```python
from build123d import *

# Parameters (mm, degrees)
CYLINDER001_R              = 1.5
CYLINDER001_DEPTH          = 10
BOX001_W                   = 5
BOX001_H                   = 2
BOX001_DEPTH               = 5
BOX_W                      = 5
BOX_H                      = 5
BOX_DEPTH                  = 10
FILLET_R                   = 2
FILLET_PLACEMENT_ANGLE     = 90
CHAMFER_SIZE               = 4
SKETCH005_R                = 54
SKETCH005_R_2              = 48.75
PAD003_DEPTH               = 1.5
SKETCH006_R                = 1.5
POCKET002_DEPTH            = 1.501
CYLINDER003_R              = 1.5
CYLINDER003_DEPTH          = 10
BOX005_W                   = 5
BOX005_H                   = 2
BOX005_DEPTH               = 5
BOX004_W                   = 5
BOX004_H                   = 5
BOX004_DEPTH               = 10
FILLET002_R                = 2
FILLET002_PLACEMENT_ANGLE  = 90
CHAMFER002_SIZE            = 4
CHAMFER002_PLACEMENT_ANGLE = 90
CYLINDER004_R              = 1.5
CYLINDER004_DEPTH          = 10
BOX007_W                   = 5
BOX007_H                   = 2
BOX007_DEPTH               = 5
BOX006_W                   = 5
BOX006_H                   = 5
BOX006_DEPTH               = 10
FILLET003_R                = 2
FILLET003_PLACEMENT_ANGLE  = 90
CHAMFER003_SIZE            = 4
CHAMFER003_PLACEMENT_ANGLE = 180
CYLINDER005_R              = 1.5
CYLINDER005_DEPTH          = 10
BOX009_W                   = 5
BOX009_H                   = 2
BOX009_DEPTH               = 5
BOX008_W                   = 5
BOX008_H                   = 5
BOX008_DEPTH               = 10
FILLET004_R                = 2
FILLET004_PLACEMENT_ANGLE  = 90
CHAMFER004_SIZE            = 4
CHAMFER004_PLACEMENT_ANGLE = 90


with BuildPart() as screw:
    # Cylinder001 → Cylinder001 (new body)
    with BuildSketch(Plane(origin=(2.5, -2.75, 7.5), x_dir=(0, 0, 1), z_dir=(0, 1, 0))):
        Circle(CYLINDER001_R)
    extrude(amount=CYLINDER001_DEPTH)


with BuildPart() as extleghole:
    # Box001 → Box001 (new body)
    with BuildSketch(Plane(origin=(0, 1.5, 5), x_dir=(1, 0, 0), z_dir=(0, 0, 1))):
        with Locations((2.5, 1)):
            Rectangle(BOX001_W, BOX001_H)
    extrude(amount=BOX001_DEPTH)


with BuildPart() as screwext:
    # Box → Box (new body)
    with BuildSketch(Plane.XY):
        with Locations((2.5, 2.5)):
            Rectangle(BOX_W, BOX_H)
    extrude(amount=BOX_DEPTH)

    # Cut: cut ExtLegHole
    add(extleghole.part, mode=Mode.SUBTRACT)

    # Cut001: cut Screw
    add(screw.part, mode=Mode.SUBTRACT)

    # Fillet
    fillet_edges = [screwext.edges().sort_by_distance(p)[0] for p in [
        (0, 0.75, 10),
        (0, 4.25, 10),
        (5, 0.75, 10),
        (5, 4.25, 10),
    ]]
    fillet(fillet_edges, radius=FILLET_R)


with BuildPart() as screwext_1:
    # Fillet placement: moved
    add(screwext.part.moved(Location((49, -2.5, 5))).rotate(Axis((49, -2.5, 5), (0, 1, 0)), FILLET_PLACEMENT_ANGLE))

    # Chamfer
    chamfer_edges = [screwext_1.edges().sort_by_distance(p)[0] for p in [
        (49, 0, 5),
    ]]
    chamfer(chamfer_edges, length=CHAMFER_SIZE)


with BuildPart() as fusion:
    # Sketch005 → Pad003 (new body)
    with BuildSketch(Plane.XY):
        Circle(SKETCH005_R)
        Circle(SKETCH005_R_2, mode=Mode.SUBTRACT)
    extrude(amount=PAD003_DEPTH)

    # Sketch006 (on Face4 of Pad003) → Pocket002 (cut, through all)
    with BuildSketch(Plane.XY.offset(1.5)):
        with Locations((46, 22.5)):
            Circle(SKETCH006_R)
        with Locations((-46, -22.5)):
            Circle(SKETCH006_R)
        with Locations((-46, 22.5)):
            Circle(SKETCH006_R)
        with Locations((46, -22.5)):
            Circle(SKETCH006_R)
    extrude(amount=-POCKET002_DEPTH, mode=Mode.SUBTRACT)

    # Fusion: union ScrewExt
    add(screwext_1.part)


with BuildPart() as screw002:
    # Cylinder003 → Cylinder003 (new body)
    with BuildSketch(Plane(origin=(2.5, -2.75, 7.5), x_dir=(0, 0, 1), z_dir=(0, 1, 0))):
        Circle(CYLINDER003_R)
    extrude(amount=CYLINDER003_DEPTH)


with BuildPart() as extleghole002:
    # Box005 → Box005 (new body)
    with BuildSketch(Plane(origin=(0, 1.5, 5), x_dir=(1, 0, 0), z_dir=(0, 0, 1))):
        with Locations((2.5, 1)):
            Rectangle(BOX005_W, BOX005_H)
    extrude(amount=BOX005_DEPTH)


with BuildPart() as fusion001:
    # Box004 → Box004 (new body)
    with BuildSketch(Plane.XY):
        with Locations((2.5, 2.5)):
            Rectangle(BOX004_W, BOX004_H)
    extrude(amount=BOX004_DEPTH)

    # Cut004: cut ExtLegHole002
    add(extleghole002.part, mode=Mode.SUBTRACT)

    # Cut005: cut Screw002
    add(screw002.part, mode=Mode.SUBTRACT)

    # Fillet002
    fillet002_edges = [fusion001.edges().sort_by_distance(p)[0] for p in [
        (0, 0.75, 10),
        (0, 4.25, 10),
        (5, 0.75, 10),
        (5, 4.25, 10),
    ]]
    fillet(fillet002_edges, radius=FILLET002_R)


with BuildPart() as fusion001_1:
    # Fillet002 placement: moved
    add(fusion001.part.moved(Location((49, -2.5, 5))).rotate(Axis((49, -2.5, 5), (0, 1, 0)), FILLET002_PLACEMENT_ANGLE))

    # Chamfer002
    chamfer002_edges = [fusion001_1.edges().sort_by_distance(p)[0] for p in [
        (49, 0, 5),
    ]]
    chamfer(chamfer002_edges, length=CHAMFER002_SIZE)


with BuildPart() as fusion001_2:
    # Chamfer002 placement: moved
    add(fusion001_1.part.rotate(Axis((0, 0, 0), (0, 0, 1)), CHAMFER002_PLACEMENT_ANGLE))

    # Fusion001: union Fusion
    add(fusion.part)


with BuildPart() as screw003:
    # Cylinder004 → Cylinder004 (new body)
    with BuildSketch(Plane(origin=(2.5, -2.75, 7.5), x_dir=(0, 0, 1), z_dir=(0, 1, 0))):
        Circle(CYLINDER004_R)
    extrude(amount=CYLINDER004_DEPTH)


with BuildPart() as extleghole003:
    # Box007 → Box007 (new body)
    with BuildSketch(Plane(origin=(0, 1.5, 5), x_dir=(1, 0, 0), z_dir=(0, 0, 1))):
        with Locations((2.5, 1)):
            Rectangle(BOX007_W, BOX007_H)
    extrude(amount=BOX007_DEPTH)


with BuildPart() as fusion002:
    # Box006 → Box006 (new body)
    with BuildSketch(Plane.XY):
        with Locations((2.5, 2.5)):
            Rectangle(BOX006_W, BOX006_H)
    extrude(amount=BOX006_DEPTH)

    # Cut006: cut ExtLegHole003
    add(extleghole003.part, mode=Mode.SUBTRACT)

    # Cut007: cut Screw003
    add(screw003.part, mode=Mode.SUBTRACT)

    # Fillet003
    fillet003_edges = [fusion002.edges().sort_by_distance(p)[0] for p in [
        (0, 0.75, 10),
        (0, 4.25, 10),
        (5, 0.75, 10),
        (5, 4.25, 10),
    ]]
    fillet(fillet003_edges, radius=FILLET003_R)


with BuildPart() as fusion002_1:
    # Fillet003 placement: moved
    add(fusion002.part.moved(Location((49, -2.5, 5))).rotate(Axis((49, -2.5, 5), (0, 1, 0)), FILLET003_PLACEMENT_ANGLE))

    # Chamfer003
    chamfer003_edges = [fusion002_1.edges().sort_by_distance(p)[0] for p in [
        (49, 0, 5),
    ]]
    chamfer(chamfer003_edges, length=CHAMFER003_SIZE)


with BuildPart() as fusion002_2:
    # Chamfer003 placement: moved
    add(fusion002_1.part.rotate(Axis((0, 0, 0), (0, 0, 1)), CHAMFER003_PLACEMENT_ANGLE))

    # Fusion002: union Fusion001
    add(fusion001_2.part)


with BuildPart() as screw004:
    # Cylinder005 → Cylinder005 (new body)
    with BuildSketch(Plane(origin=(2.5, -2.75, 7.5), x_dir=(0, 0, 1), z_dir=(0, 1, 0))):
        Circle(CYLINDER005_R)
    extrude(amount=CYLINDER005_DEPTH)


with BuildPart() as extleghole004:
    # Box009 → Box009 (new body)
    with BuildSketch(Plane(origin=(0, 1.5, 5), x_dir=(1, 0, 0), z_dir=(0, 0, 1))):
        with Locations((2.5, 1)):
            Rectangle(BOX009_W, BOX009_H)
    extrude(amount=BOX009_DEPTH)


with BuildPart() as obj1:
    # Box008 → Box008 (new body)
    with BuildSketch(Plane.XY):
        with Locations((2.5, 2.5)):
            Rectangle(BOX008_W, BOX008_H)
    extrude(amount=BOX008_DEPTH)

    # Cut008: cut ExtLegHole004
    add(extleghole004.part, mode=Mode.SUBTRACT)

    # Cut009: cut Screw004
    add(screw004.part, mode=Mode.SUBTRACT)

    # Fillet004
    fillet004_edges = [obj1.edges().sort_by_distance(p)[0] for p in [
        (0, 0.75, 10),
        (0, 4.25, 10),
        (5, 0.75, 10),
        (5, 4.25, 10),
    ]]
    fillet(fillet004_edges, radius=FILLET004_R)


with BuildPart() as obj1_1:
    # Fillet004 placement: moved
    add(obj1.part.moved(Location((49, -2.5, 5))).rotate(Axis((49, -2.5, 5), (0, 1, 0)), FILLET004_PLACEMENT_ANGLE))

    # Chamfer004
    chamfer004_edges = [obj1_1.edges().sort_by_distance(p)[0] for p in [
        (49, 0, 5),
    ]]
    chamfer(chamfer004_edges, length=CHAMFER004_SIZE)


with BuildPart() as obj1_2:
    # Chamfer004 placement: moved
    add(obj1_1.part.rotate(Axis((0, 0, 0), (0, 0, -1)), CHAMFER004_PLACEMENT_ANGLE))

    # Fusion003: union Fusion002
    add(fusion002_2.part)


solid = obj1_2.part
```
Verification items for the finished model (mm, model axes). A direction names the side the tool comes from. Give positions to 0.01 mm unless a question says otherwise; leave off trailing zeros. Order: outer loops, then holes, each group sorted by start corner. A loop starts at its lowest first (then second) coordinate and runs counter-clockwise, first axis right, second up. Notation, with made-up numbers: M 12.25,-24.75 L 60.25,-24.75 A21 cw 60.25,-12.75 Z; hole C -15,72 d7. An arc over 180 degrees is marked long. Answer in a Markdown table with one row per item. Add a question column.
Item 1: Gauge pin test, flat ends, axial feed: pin 1 (1.8 mm diameter, centred on y = 56.5, z = 2.5, fed in from +X); pin 2 (1.5 mm diameter, centred on y = 55.5, z = 3.5, fed in from -X); pin 3 (2.5 mm diameter, centred on y = 56, z = 1.5, fed in from +X); pin 4 (5 mm diameter, centred on x = -46, y = -22.5, fed in from +Z). Record the tip position at first contact, or that the pin passes through.
Item 2: Tool access check on faces 1 (the flat face through (2.5, -54, 3)), 2 (the flat face through (-54, 2.5, 3)), 3 (the flat face through (0, 51, 3)), 4 (the flat face through (1, 55, 1)), 5 (the flat face through (-55, 1, 1)). Record the directions out of +Z, -Z, +X, -X, +Y, -Y that give a thin tool (end or side, any length) a straight path to the whole face; none if there is none.
Item 3: Scan lines: probe 1 along Z at (x, y) = (-56.5, -1.75); probe 2 along X at (y, z) = (11.5, 0.85); probe 3 along Y at (x, z) = (22.5, 0.8). Record each from-to range of solid material in increasing order. Write a range as from..to.
Item 4: Mould release check, pull along X, two halves, no side actions. Record for faces 6 (the flat face through (54, -2.5, 3)), 7 (the cylindrical face through (44.5, -22.43, 0.76)), 8 (the flat face through (2.5, 54, 3)): released by +X, released by -X, zero draft, split by the parting line, or undercut.
Item 5: Section check C-C, the plane x = -33.5. Enter the section's corners in (y, z), and give its area (3 significant figures).
Item 6: Section check A-A, the plane y = -6.5. Enter the section's corners in (x, z), and give its area (3 significant figures).
Item 7: Section check B-B, the plane x = 46. Enter the section's corners in (y, z).
Item 8: Section check D-D, the plane y = -22.5. Enter the section's corners in (x, z), and give its area (3 significant figures).
Filled sheet:
| question | item | result |
|---|---|---|
| 1 | pin 1 | passes through |
| 1 | pin 2 | stops at x = -2.5 |
| 1 | pin 3 | stops at x = 2.5 |
| 1 | pin 4 | stops at z = 1.5 |
| 2 | face 1 | +Z, +X, -Y |
| 2 | face 2 | +Z, -X, +Y |
| 2 | face 3 | +Z, +X, -X |
| 2 | face 4 | +Z, -Z, +Y |
| 2 | face 5 | +Z, -Z, -X |
| 3 | probe 1 | z = 0..1, 4..5 |
| 3 | probe 2 | x = -52.76..-47.37, 47.37..52.76 |
| 3 | probe 3 | y = -49.09..-43.25, 43.25..49.09 |
| 4 | face 6 | zero draft |
| 4 | face 7 | undercut |
| 4 | face 8 | released by +X |
| 5 | outline | M -42.35,0 L -35.42,0 L -35.42,1.5 L -42.35,1.5 Z; M 35.42,0 L 42.35,0 L 42.35,1.5 L 35.42,1.5 Z |
| 5 | area | 20.8 mm^2 |
| 6 | outline | M -53.61,0 L -48.31,0 L -48.31,1.5 L -53.61,1.5 Z; M 48.31,0 L 53.61,0 L 53.61,1.5 L 48.31,1.5 Z |
| 6 | area | 15.9 mm^2 |
| 7 | outline | M -28.28,0 L -24,0 L -24,1.5 L -28.28,1.5 Z; M -21,0 L -16.14,0 L -16.14,1.5 L -21,1.5 Z; M 16.14,0 L 21,0 L 21,1.5 L 16.14,1.5 Z; M 24,0 L 28.28,0 L 28.28,1.5 L 24,1.5 Z |
| 8 | outline | M -49.09,0 L -47.5,0 L -47.5,1.5 L -49.09,1.5 Z; M -44.5,0 L -43.25,0 L -43.25,1.5 L -44.5,1.5 Z; M 43.25,0 L 44.5,0 L 44.5,1.5 L 43.25,1.5 Z; M 47.5,0 L 49.09,0 L 49.09,1.5 L 47.5,1.5 Z |
| 8 | area | 8.53 mm^2 |
